Geometry: final body of the model. Coordinates: model frame, mm. Face numbers are marked on the shaded views. A direction names the side the tool comes from. Give positions to 0.01 mm unless a question says otherwise; leave off trailing zeros. Write each loop counter-clockwise with the first axis right and the second up, starting at its lowest first coordinate (ties: lowest second). Pieces come first, ordered by that corner, then holes.
from build123d import *

# Parameters (mm, degrees)
SKETCH1_W           = 60
SKETCH1_H           = 40
SKETCH1_W_2         = 19
SKETCH1_H_2         = 15
BOSS_EXTRUDE1_DEPTH = 20
SHELL2_T            = -3
SKETCH1_3_W         = 19
SKETCH1_3_H         = 15
BOSS_EXTRUDE2_DEPTH = 3
SKETCH2_W           = 20
SKETCH2_H           = 17
CUT_EXTRUDE1_DEPTH  = 3
CHAMFER1_SIZE       = 3
BOSS_EXTRUDE3_REACH = 53.662


with BuildPart() as part:
    # Sketch1 → Boss-Extrude1 (new body)
    # profile 1 of 2: a face of its own
    with BuildSketch(Plane(origin=(0, 0, 0), x_dir=(1, 0, 0), z_dir=(0, 1, 0))):
        Rectangle(SKETCH1_W, SKETCH1_H)
        Rectangle(SKETCH1_W_2, SKETCH1_H_2, mode=Mode.SUBTRACT)
    # profile 2 of 2: a face of its own
    with BuildSketch(Plane(origin=(0, 0, 0), x_dir=(1, 0, 0), z_dir=(0, 1, 0))):
        Rectangle(SKETCH1_W_2, SKETCH1_H_2)
    extrude(amount=BOSS_EXTRUDE1_DEPTH)

    # Shell2
    shell2_openings = [part.faces().sort_by_distance(p)[0] for p in [
        (0, 20, 0),
    ]]
    offset(amount=SHELL2_T, openings=shell2_openings, kind=Kind.INTERSECTION)

    # Sketch1<3> → Boss-Extrude2 (add)
    with BuildSketch(Plane(origin=(0, 0, 0), x_dir=(1, 0, 0), z_dir=(0, 1, 0))):
        Rectangle(SKETCH1_3_W, SKETCH1_3_H)
    extrude(amount=-BOSS_EXTRUDE2_DEPTH)

    # Sketch2 → Cut-Extrude1 (cut)
    with BuildSketch(Plane(origin=(30, 0, 0), x_dir=(0, 0, -1), z_dir=(1, 0, 0))):
        with Locations((0, 11.5)):
            Rectangle(SKETCH2_W, SKETCH2_H)
    extrude(amount=-CUT_EXTRUDE1_DEPTH, mode=Mode.SUBTRACT)

    # Chamfer1
    chamfer1_edges = [part.edges().sort_by_distance(p)[0] for p in [
        (30, 3, 0),
    ]]
    chamfer(chamfer1_edges, length=CHAMFER1_SIZE - 0.0001)  # a hair under: the kernel refuses the full size

    # Sketch3 → Boss-Extrude3 (add, up to next)
    with BuildSketch(Plane.XY.offset(-17), mode=Mode.PRIVATE) as boss_extrude3_sk1:
        Polygon((-27, 3), (27, 3), (-27, 12.521656958), align=None)
    boss_extrude3_tool1 = extrude(boss_extrude3_sk1.sketch, amount=BOSS_EXTRUDE3_REACH, mode=Mode.PRIVATE) - part.part
    add(boss_extrude3_tool1.solids().sort_by_distance((-9, 6.173886, -17))[0])


solid = part.part
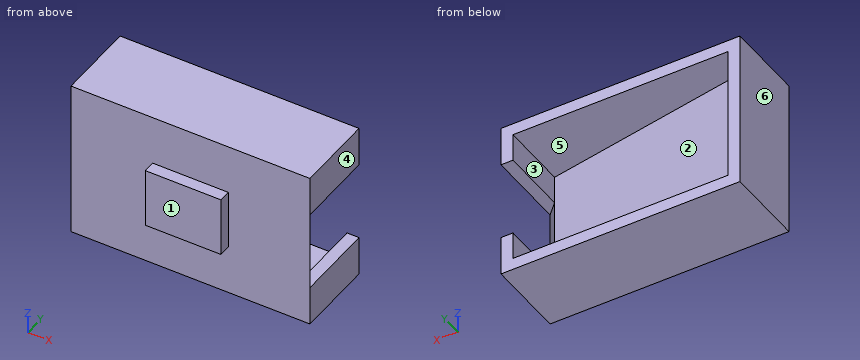
Q1. Pin query (flat end, axial travel): P1, Ø0.9, axis at x = 2.5, y = -2, coming from the +Z side; P2, Ø2, axis at y = 17.5, z = 5.5, coming from the +X side; P3, Ø3.5, axis at x = 0, y = -2, coming from the -Z side. Return the tip coordinate at first contact, or that it passes through.
Filled sheet:
P1: stops at z = 7.5
P2: stops at x = -27
P3: stops at z = -7.5
Q2. Section C-C on z = 14.5. Output: boundary loops of the cut face in (x, y).
Filled sheet:
outline: (-30, 0) - (30, 0) - (30, 20) - (27, 20) - (27, 3) - (-27, 12.52) - (-27, 20) - (-30, 20) - close
Q3. Section D-D on x = -12. Output: boundary loops of the cut face in (y, z), plus the area to 3 significant figures.
Filled sheet:
outline: (0, -20) - (20, -20) - (20, -17) - (9.88, -17) - (9.88, 17) - (20, 17) - (20, 20) - (0, 20) - close
area: 456 mm2
Q4. Ray query, line 1 along X through (y, z) = (15.5, 15); line 2 along Z through (x, y) = (1, 10.25); line 3 along Y through (x, z) = (-3.5, -17.5). Return the intervals inside material, ascending.
Filled sheet:
line 1: x = -30 to -27, 27 to 30
line 2: z = -20 to -17, 17 to 20
line 3: y = 0 to 20
Q5. Pull-direction query (X, two-part tool) for the marked faces 3, 4, 5 and 6; classes: released by +X, released by -X, zero draft, split by the parting line, or undercut.
Filled sheet:
face 3: undercut
face 4: released by +X
face 5: undercut
face 6: released by -X
Q6. Access query for the marked faces 1 and 2. Directions: +Z, -Z, +X, -X, +Y, -Y. A direction counts if a zero-diameter tool reaches every point of the face in a straight line with its end or side. Return the directions, or none.
Filled sheet:
face 1: +Z, -Z, +X, -X, -Y
face 2: +Y
Q7. Section A-A on y = 17.5. Output: boundary loops of the cut face in (x, z), plus the area to 3 significant figures.
Filled sheet:
outline: (-30, -20) - (30, -20) - (30, -10) - (27, -10) - (27, -17) - (-27, -17) - (-27, 17) - (27, 17) - (27, 10) - (30, 10) - (30, 20) - (-30, 20) - close
area: 504 mm2
Q8. Section B-B on x = 3. Output: boundary loops of the cut face in (y, z), plus the area to 3 significant figures.
Filled sheet:
outline: (-3, -7.5) - (0, -7.5) - (0, -20) - (20, -20) - (20, -17) - (7.23, -17) - (7.23, 17) - (20, 17) - (20, 20) - (0, 20) - (0, 7.5) - (-3, 7.5) - close
area: 411 mm2
